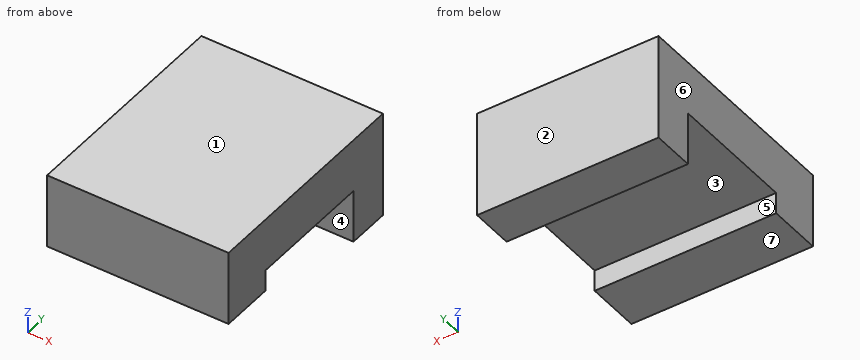
```python
from build123d import *

# Parameters (mm, degrees)
F0_W     = 17
F0_H     = 4
F1_DEPTH = 10
F2_W     = 17
F2_H     = 5
F3_DEPTH = 12
F4_W     = 17
F4_H     = 7
F5_DEPTH = 5


with BuildPart() as f1:
    # F0 (on Top) → F1 (new body)
    with BuildSketch(Plane.XY):
        with Locations((5.519233, -6.434065)):
            Rectangle(F0_W, F0_H)
    extrude(amount=F1_DEPTH)

    # F2 (on face) → F3 (join)
    with BuildSketch(Plane.XZ.offset(8.434065)):
        with Locations((5.519233, 7.5)):
            Rectangle(F2_W, F2_H)
    extrude(amount=F3_DEPTH)

    # F4 (on face) → F5 (join)
    with BuildSketch(Plane.XZ.offset(20.434065)):
        with Locations((5.519233, 6.5)):
            Rectangle(F4_W, F4_H)
    extrude(amount=F5_DEPTH)


solid = f1.part
```
Could you check a few things on this model? Use its own coordinates, in mm. Face numbers are marked on the shaded views. A direction names the side the tool comes from. Round coordinates to 2 decimals unless told otherwise and drop trailing zeros. Order: outer loops, then holes, each group sorted by start corner. A loop starts at its lowest first (then second) coordinate and runs counter-clockwise, first axis right, second up. Notation, with made-up numbers: M 72.25,69 L 89.25,69 A8 cw 89.25,82 Z; hole C -22,-26.75 d10. An arc over 180 degrees is marked long. One line per question, with ' | ' between items. Start each with the question number.
(1) Suppose I cut it at D-D on z = 1.5. List the corners of the cut face in (x, y) for me, then the cut area to 3 significant figures.
(2) For the marked faces 5, 6 and 7, which set-ups out of +Z, -Z, +X, -X, +Y, -Y let a thin tool reach every point of the face, with its end or its side?
(3) Suppose I cut it at A-A on z = 3.75. List the corners of the cut face in (x, y) for me, then the cut area to 3 significant figures.
(4) For P1, Ø2, axis at y = -10.5, z = 2.5, coming from the -X side; P2, Ø9.5, axis at x = 2, y = -14.5, coming from the -Z side; P3, Ø2.5, axis at x = 8, y = -22, coming from the -Z side, each with a flat end and sliding along its axis, tell me the tip position at first contact or that it passes through.
(5) Suppose I cut it at B-B on x = 4.5. List the corners of the cut face in (y, z) for me, then the cut area to 3 significant figures.
(6) Suppose I cut it at C-C on y = -10.5. List the corners of the cut face in (x, z) for me, then the cut area to 3 significant figures.
(7) Please list where these lines run through material, in increasing order: line 1 along Y through (x, z) = (9, 4.5); line 2 along Z through (x, y) = (5.25, -11.25); line 3 along Y through (x, z) = (1, 0.5).
(8) Thinking about a two-plate mould opening in Y: for the marked faces 1, 2, 3 and 4, which applies, +Y half, -Y half, draft (parallel to the pull), parting line (faces both ways), or undercut?
Geometry results:
1) outline: M -2.98,-8.43 L 14.02,-8.43 L 14.02,-4.43 L -2.98,-4.43 Z | area: 68.0 mm²
2) face 5: -Z, +X, -X | face 6: +Z, -Z, -X, +Y, -Y | face 7: -Z, +X, -X, -Y
3) outline: M -2.98,-25.43 L 14.02,-25.43 L 14.02,-20.43 L -2.98,-20.43 Z; M -2.98,-8.43 L 14.02,-8.43 L 14.02,-4.43 L -2.98,-4.43 Z | area: 153 mm²
4) P1: through | P2: z = 5 | P3: z = 3
5) outline: M -25.43,3 L -20.43,3 L -20.43,5 L -8.43,5 L -8.43,0 L -4.43,0 L -4.43,10 L -25.43,10 Z | area: 135 mm²
6) outline: M -2.98,5 L 14.02,5 L 14.02,10 L -2.98,10 Z | area: 85.0 mm²
7) line 1: -25.43 to -20.43, -8.43 to -4.43 | line 2: 5 to 10 | line 3: -8.43 to -4.43
8) face 1: draft | face 2: +Y half | face 3: undercut | face 4: undercut
